from build123d import *

# Parameters (mm, degrees)
PAD010_DEPTH    = 125
CHAMFER003_SIZE = 20
FILLET007_R     = 5


with BuildPart() as part:
    # Sketch014 → Pad010 (new body)
    with BuildSketch(Plane.XZ.offset(-215)):
        with BuildLine():
            Line((397.8, 325), (232.8, 325))
            Line((232.8, 325), (232.8, 240))
            ThreePointArc((303.474182, 126.999993), (284.350647, 193.640525), (232.8, 240))
            Line((303.474182, 61.999993), (303.474182, 126.999993))
            Line((397.8, 115), (303.474182, 61.999993))
            Line((397.8, 325), (397.8, 115))
        make_face()
    extrude(amount=-PAD010_DEPTH)

    # Chamfer003
    chamfer003_edges = [part.edges().sort_by_distance(p)[0] for p in [
        (315.3, 340, 325),
    ]]
    chamfer(chamfer003_edges, length=CHAMFER003_SIZE)

    # Fillet007
    fillet007_edges = [part.edges().sort_by_distance(p)[0] for p in [
        (397.8, 340, 210),
        (397.8, 277.5, 115),
        (350.637091, 340, 88.499996),
        (303.474182, 340, 94.499993),
        (284.350647, 340, 193.640525),
        (232.8, 340, 272.5),
        (397.8, 215, 220),
        (350.637091, 215, 88.499996),
        (303.474182, 277.5, 61.999993),
    ]]
    fillet(fillet007_edges, radius=FILLET007_R)


solid = part.part
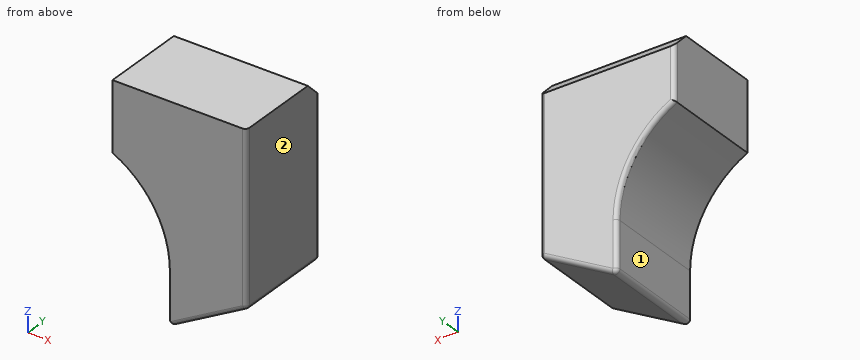
Work out the finished part from the listing and answer in its coordinate system (mm). Face numbers are marked on the shaded views. A direction names the side the tool comes from. Coordinates: 2 decimals unless noted, no trailing zeros. Write each loop counter-clockwise with the first axis right and the second up, starting at its lowest first coordinate (ties: lowest second). Pieces come first, ordered by that corner, then holes. Notation, with made-up numbers: M 63,15 L 96,15 A19 cw 96,27 Z; hole C 72.25,19 d2. An arc over 180 degrees is marked long. Answer as CSV lines item,"result". Start each with the question number.
Item 1: Flat-ended cylindrical pins translate along their axes: P1, Ø17, axis at y = 250.5, z = 113, coming from the -X side; P2, Ø1.5, axis at x = 335.5, y = 278, coming from the -Z side; P3, Ø10, axis at x = 269.5, y = 243, coming from the -Z side. Find the tip coordinate at first contact, or state that the pin passes through.
Item 2: Section A-A on y = 241 is taken. Write down the section's boundary in (x, z).
Item 3: A tool of negligible diameter and unlimited length cuts with its end or side. For the marked faces 1 and 2, from which of +Z, -Z, +X, -X, +Y, -Y can it reach the whole face along a straight path? Write none if from no direction.
Item 4: Consider L1, parallel to X at y = 245, z = 177; L2, parallel to Z at x = 327.5, y = 243.5; L3, parallel to X at y = 274, z = 182. Determine where each line is inside the solid, lowest interval first.
Checks:
1,P1,"stops at x = 303.47"
1,P2,"stops at z = 79.57"
1,P3,"stops at z = 207.27"
2,outline,"M 232.8,240 A125.67 cw 303.47,127 L 303.47,70.54 A5 ccw 310.92,66.19 L 395.25,113.57 A5 ccw 397.8,117.93 L 397.8,325 L 232.8,325 Z"
3,face 1,"-Z, -X, +Y, -Y"
3,face 2,"+Z, -Z, +X, +Y, -Y"
4,L1,"x = 293.1 to 397.8"
4,L2,"z = 75.5 to 325"
4,L3,"x = 290.8 to 397.8"
